Input: part model. Units: mm. Frame: model coordinates. Face numbers are marked on the shaded views. Round coordinates to 2 decimals unless told otherwise and drop trailing zeros. Loops run counter-clockwise (first coordinate to the right, second up) from the corner with the lowest first, then second, coordinate; pieces in that order, holes last.
1) First-contact query: pin 1 (5.5 mm diameter, centred on x = -103, z = 0, fed in from +Y); pin 2 (1 mm diameter, centred on x = 9.5, y = 9.5, fed in from -Z); pin 3 (10 mm diameter, centred on x = -21, z = 46, fed in from +Y); pin 4 (4 mm diameter, centred on x = 103, z = 0, fed in from +Y). Flat tips, straight axial feed; report the tip coordinate or a pass-through.
2) Section B-B, the plane x = 5. Return loops of the section in (y, z), and give its area (3 significant figures).
3) Section D-D, the plane x = 50. Return loops of the section in (y, z).
4) Draft query along Z for the marked faces 1 and 2. Return one class per face: pulls with the +Z half, pulls with the -Z half, needs draft (parallel to the pull), parting line crosses it, or undercut.
5) Section A-A, the plane y = 6.5. Return loops of the section in (x, z).
6) Ray query, line 1 along X through (y, z) = (0.5, 0.5); line 2 along Z through (x, y) = (0, 9); line 3 along Z through (x, y) = (-1, 2.75). Return the intervals inside material, ascending.
7) Section C-C, the plane z = -83. Return loops of the section in (x, y), and give its area (3 significant figures).
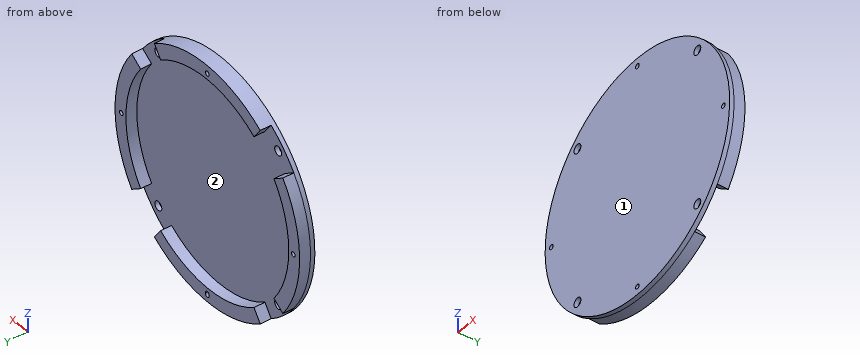
from build123d import *

# Parameters (mm, degrees)
SCHIZZO1_R                       = 110.5
SCHIZZO1_R_2                     = 2.15
SCHIZZO1_R_3                     = 4.15
ESTRUSIONE_ESTRUSIONE1_DEPTH     = 4
ESTRUSIONE_ESTRUSIONE2_OUTLINE_R = 2.15
ESTRUSIONE_ESTRUSIONE2_DEPTH     = 10


# Read off the part's stored shape, not the designer's step: Estrusione-Estrusione2
with BuildPart() as part:
    # Schizzo1 → Estrusione-Estrusione1 (new body)
    with BuildSketch(Plane(origin=(0, 0, 0), x_dir=(1, 0, 0), z_dir=(0, 1, 0))):
        with Locations(Location((0, 0, 0), (0, 0, 270))):
            Circle(SCHIZZO1_R)
        with Locations(Location((-103, 0, 0), (0, 0, 270))):
            Circle(SCHIZZO1_R_2, mode=Mode.SUBTRACT)
        with Locations(Location((0, 103, 0), (0, 0, 270))):
            Circle(SCHIZZO1_R_2, mode=Mode.SUBTRACT)
        with Locations(Location((103, 0, 0), (0, 0, 270))):
            Circle(SCHIZZO1_R_2, mode=Mode.SUBTRACT)
        with Locations(Location((0, -103, 0), (0, 0, 270))):
            Circle(SCHIZZO1_R_2, mode=Mode.SUBTRACT)
        with Locations(Location((-71.77133829, 71.77133829, 0), (0, 0, 270))):
            Circle(SCHIZZO1_R_3, mode=Mode.SUBTRACT)
        with Locations(Location((71.77133829, 71.77133829, 0), (0, 0, 270))):
            Circle(SCHIZZO1_R_3, mode=Mode.SUBTRACT)
        with Locations(Location((71.77133829, -71.77133829, 0), (0, 0, 270))):
            Circle(SCHIZZO1_R_3, mode=Mode.SUBTRACT)
        with Locations(Location((-71.77133829, -71.77133829, 0), (0, 0, 270))):
            Circle(SCHIZZO1_R_3, mode=Mode.SUBTRACT)
    extrude(amount=ESTRUSIONE_ESTRUSIONE1_DEPTH)

    # Estrusione-Estrusione2 outline → Estrusione-Estrusione2 (add)
    # profile 1 of 4: a face of its own
    with BuildSketch(Plane(origin=(0, 4, 0), x_dir=(1, 0, 0), z_dir=(0, 1, 0))):
        with BuildLine():
            ThreePointArc((90.516300894, -63.380196217), (110.5, 0), (90.516300894, 63.380196217))
            Line((90.516300894, 63.380196217), (79.867324318, 55.923702544))
            ThreePointArc((79.867324318, 55.923702544), (97.5, 0), (79.867324318, -55.923702544))
            Line((79.867324318, -55.923702544), (90.516300894, -63.380196217))
        make_face()
        with Locations((103, 0)):
            Circle(ESTRUSIONE_ESTRUSIONE2_OUTLINE_R, mode=Mode.SUBTRACT)
    # profile 2 of 4: a face of its own
    with BuildSketch(Plane(origin=(0, 4, 0), x_dir=(1, 0, 0), z_dir=(0, 1, 0))):
        with BuildLine():
            Line((55.923702544, 79.867324318), (63.380196217, 90.516300894))
            ThreePointArc((63.380196217, 90.516300894), (0, 110.5), (-63.380196217, 90.516300894))
            Line((-63.380196217, 90.516300894), (-55.923702544, 79.867324318))
            ThreePointArc((-55.923702544, 79.867324318), (0, 97.5), (55.923702544, 79.867324318))
        make_face()
        with BuildLine():
            ThreePointArc((2.091052367, 103.5), (0, 100.85), (-2.091052367, 103.5))
            ThreePointArc((-2.091052367, 103.5), (0, 106.15), (2.091052367, 103.5))
        make_face(mode=Mode.SUBTRACT)
    # profile 3 of 4: a face of its own
    with BuildSketch(Plane(origin=(0, 4, 0), x_dir=(1, 0, 0), z_dir=(0, 1, 0))):
        with BuildLine():
            ThreePointArc((-63.380196217, -90.516300894), (0, -110.5), (63.380196217, -90.516300894))
            Line((63.380196217, -90.516300894), (55.923702544, -79.867324318))
            ThreePointArc((55.923702544, -79.867324318), (0, -97.5), (-55.923702544, -79.867324318))
            Line((-55.923702544, -79.867324318), (-63.380196217, -90.516300894))
        make_face()
        with Locations((0, -103)):
            Circle(ESTRUSIONE_ESTRUSIONE2_OUTLINE_R, mode=Mode.SUBTRACT)
    # profile 4 of 4: a face of its own
    with BuildSketch(Plane(origin=(0, 4, 0), x_dir=(1, 0, 0), z_dir=(0, 1, 0))):
        with BuildLine():
            Line((-79.867324318, 55.923702544), (-90.516300894, 63.380196217))
            ThreePointArc((-90.516300894, 63.380196217), (-110.5, 0), (-90.516300894, -63.380196217))
            Line((-90.516300894, -63.380196217), (-79.867324318, -55.923702544))
            ThreePointArc((-79.867324318, -55.923702544), (-97.5, 0), (-79.867324318, 55.923702544))
        make_face()
        with Locations((-103, 0)):
            Circle(ESTRUSIONE_ESTRUSIONE2_OUTLINE_R, mode=Mode.SUBTRACT)
    extrude(amount=ESTRUSIONE_ESTRUSIONE2_DEPTH)


solid = part.part
Final values:
1. pin 1: stops at y = 14
1. pin 2: stops at z = -110.13
1. pin 3: stops at y = 4
1. pin 4: passes through
2. outline: (0, -110.39) - (14, -110.39) - (14, -97.37) - (4, -97.37) - (4, 97.37) - (14, 97.37) - (14, 110.39) - (0, 110.39) - close
2. area: 1,140 mm2
3. outline: (0, -98.54) - (14, -98.54) - (14, -83.7) - (4, -83.7) - (4, 83.7) - (14, 83.7) - (14, 98.54) - (0, 98.54) - close
4. face 1: needs draft
4. face 2: undercut
5. outline: (-90.52, -63.38) - (-79.87, -55.92) arc R97.5 cw to (-79.87, 55.92) - (-90.52, 63.38) arc R110.5 ccw to start; (-63.38, -90.52) arc R110.5 ccw to (63.38, -90.52) - (55.92, -79.87) arc R97.5 cw to (-55.92, -79.87) - close; (-63.38, 90.52) - (-55.92, 79.87) arc R97.5 cw to (55.92, 79.87) - (63.38, 90.52) arc R110.5 ccw to start; (79.87, -55.92) - (90.52, -63.38) arc R110.5 ccw to (90.52, 63.38) - (79.87, 55.92) arc R97.5 cw to start; hole circle Ø4.3 at (-103, 0); hole circle Ø4.3 at (0, 103); hole (-2.09, -103.5) arc R2.15 ccw (long way) to (2.09, -103.5) arc R2.15 ccw (long way) to start; hole circle Ø4.3 at (103, 0)
6. line 1: x = -110.5 to -105.09, -100.91 to 100.91, 105.09 to 110.5
6. line 2: z = -110.5 to -106.15, -100.85 to -97.5, 97.5 to 100.85, 105.15 to 110.5
6. line 3: z = -110.5 to -104.9, -101.1 to 101.1, 104.9 to 110.5
7. outline: (-72.95, 0) - (72.95, 0) - (72.95, 4) - (58.12, 4) - (58.12, 14) - (51.16, 14) - (51.16, 4) - (-51.16, 4) - (-51.16, 14) - (-58.12, 14) - (-58.12, 4) - (-72.95, 4) - close
7. area: 723 mm2
